from build123d import *

# Parameters (mm, degrees)
BOSS_EXTRUDE1_DEPTH      = 5
M4_CLEARANCE_HOLE1_D     = 4.5
M4_CLEARANCE_HOLE1_DEPTH = 10
M4_CLEARANCE_HOLE1_TIP   = 1.351936393
CUT_EXTRUDE1_DEPTH       = 404.143894906


with BuildPart() as part:
    # Sketch1 → Boss-Extrude1 (new body)
    with BuildSketch(Plane.XY):
        with BuildLine():
            Line((-10, 0), (-270, 0))
            ThreePointArc((-270, 0), (-277.071067812, -2.928932188), (-280, -10))
            Line((-280, -10), (-280, -280))
            ThreePointArc((-280, -280), (-277.071067812, -287.071067812), (-270, -290))
            Line((-270, -290), (-150, -290))
            ThreePointArc((-150, -290), (-142.928932188, -287.071067812), (-140, -280))
            Line((-140, -280), (-140, -150))
            Line((-140, -150), (-10, -150))
            ThreePointArc((-10, -150), (-2.928932188, -147.071067812), (0, -140))
            Line((0, -140), (0, -10))
            ThreePointArc((0, -10), (-2.928932188, -2.928932188), (-10, 0))
        make_face()
    extrude(amount=BOSS_EXTRUDE1_DEPTH)

    # M4 Clearance Hole1
    with Locations(Plane.XY.offset(5)):
        with Locations((-130, -120), (-30, -120), (-30, -20), (-130, -20), (-117.5, -107.5), (-42.5, -107.5), (-42.5, -32.5), (-117.5, -32.5)):
            Hole(M4_CLEARANCE_HOLE1_D / 2, depth=M4_CLEARANCE_HOLE1_DEPTH)
            with Locations((0, 0, -(M4_CLEARANCE_HOLE1_DEPTH + M4_CLEARANCE_HOLE1_TIP / 2))):  # 118° drill point
                Cone(0, M4_CLEARANCE_HOLE1_D / 2, M4_CLEARANCE_HOLE1_TIP, mode=Mode.SUBTRACT)

    # Sketch4 → Cut-Extrude1 (cut, through all)
    with BuildSketch(Plane.XY.offset(5)):
        with BuildLine():
            Line((-172.5, -270), (-172.5, -180))
            ThreePointArc((-172.5, -180), (-171, -178.5), (-169.5, -180))
            Line((-169.5, -180), (-169.5, -270))
            ThreePointArc((-169.5, -270), (-171, -271.5), (-172.5, -270))
        make_face()
        with BuildLine():
            Line((-198, -270), (-198, -234.5))
            ThreePointArc((-198, -234.5), (-196.5, -233), (-195, -234.5))
            Line((-195, -234.5), (-195, -270))
            ThreePointArc((-195, -270), (-196.5, -271.5), (-198, -270))
        make_face()
        with BuildLine():
            Line((-227.5, -257.5), (-227.5, -215))
            ThreePointArc((-227.5, -215), (-226, -213.5), (-224.5, -215))
            Line((-224.5, -215), (-224.5, -257.5))
            ThreePointArc((-224.5, -257.5), (-226, -259), (-227.5, -257.5))
        make_face()
    extrude(amount=-CUT_EXTRUDE1_DEPTH, mode=Mode.SUBTRACT)


solid = part.part
Part model, mm, in its own coordinate system. Round coordinates to 2 decimals unless told otherwise and drop trailing zeros. Order: outer loops, then holes, each group sorted by start corner. A loop starts at its lowest first (then second) coordinate and runs counter-clockwise, first axis right, second up. Notation, with made-up numbers: (87.5, 9) -> (96.5, 9) arc R18 ccw to (96.5, 37) -> close; hole circle Ø1 at (-31, 38.5). An arc over 180 degrees is marked (long way). Put each result on its own line as item: value.
Q1. Band-saw the part on A-A (y = -219). Give the cut face in (x, z).
From the geometry:
outline: (-280, 0) -> (-227.5, 0) -> (-227.5, 5) -> (-280, 5) -> close; (-224.5, 0) -> (-172.5, 0) -> (-172.5, 5) -> (-224.5, 5) -> close; (-169.5, 0) -> (-140, 0) -> (-140, 5) -> (-169.5, 5) -> close
Q2. Wall check: line 1 (Y direction, x = -30, z = 2.2); line 2 (X direction, y = -269, z = 1.35); line 3 (Y direction, x = -42.5, z = 2.35). Give the ranges that are in metal, low to high. Write a range as [from, to].
From the geometry:
line 1: y = [-150, -122.25], [-117.75, -22.25], [-17.75, 0]
line 2: x = [-280, -198], [-195, -172.5], [-169.5, -140]
line 3: y = [-150, -109.75], [-105.25, -34.75], [-30.25, 0]
Q3. Band-saw the part on B-B (z = 2.9). State how many separate pieces and enclosed holes the cut face has, and give its area (3 significant figures).
From the geometry:
separate pieces: 1
enclosed holes: 11
area: 60,800 mm2
